The listing builds one solid part. Answer for the finished solid, in the listing's coordinates (mm). Face numbers are marked on the shaded views. A direction names the side the tool comes from. Round coordinates to 2 decimals unless told otherwise and drop trailing zeros. Loops run counter-clockwise (first coordinate to the right, second up) from the corner with the lowest first, then second, coordinate; pieces in that order, holes last. Notation, with made-up numbers: (42, 32) -> (54, 32) arc R19 ccw to (54, 57) -> close; hole circle Ø5 at (50, 56.25). An arc over 180 degrees is marked (long way). Answer in a Markdown table with one row per item. Add a question column.
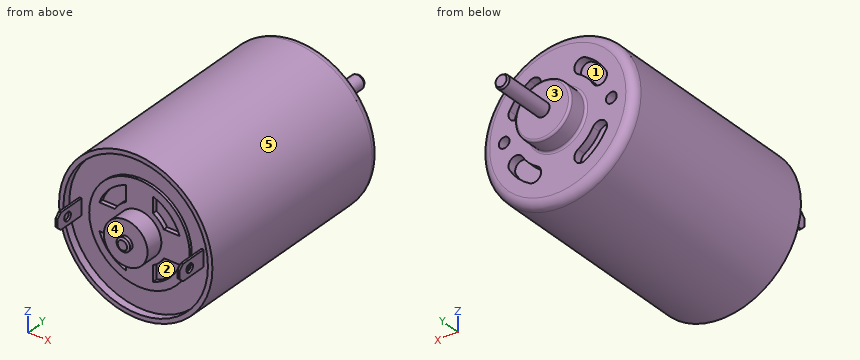
```python
from build123d import *
from OCP.BRepFilletAPI import BRepFilletAPI_MakeChamfer

# Parameters (mm, degrees)
SKETCH3_R          = 1.25
CUT_EXTRUDE2_DEPTH = 5
CUT_EXTRUDE3_DEPTH = 2
CIRPATTERN1_COUNT  = 4
CUT_EXTRUDE4_DEPTH = 1
CIRPATTERN2_COUNT  = 4
SKETCH6_W          = 3.8
SKETCH6_H          = 7.2
SKETCH6_R          = 1
EXTRUDE1_DEPTH     = 0.5
CHAMFER1_SIZE      = 1
FILLET1_R          = 2
FILLET3_R          = 0.5
CHAMFER2_SIZE      = 0.5
CHAMFER2_SIZE2     = 0.288675135


with BuildPart() as part:
    # Sketch1 → Revolve1 (revolve)
    with BuildSketch(Plane.XY, mode=Mode.PRIVATE) as revolve1_sk:
        Polygon((0, 42), (1.5875, 42), (1.5875, 29.5), (6.5, 29.5), (6.5, 25), (17.9, 25), (17.9, -25), (16.855, -25), (16.855, -23.25), (11.725, -23.25), (11.725, -23.87), (5.1, -23.87), (5.1, -28), (1.5875, -28), (1.5875, -29), (0, -29), align=None)
    revolve(revolve1_sk.sketch.rotate(Axis((0, 42, 0), (0, -1, 0)), 180), axis=Axis((0, 42, 0), (0, -1, 0)))

    # Sketch3 → Cut-Extrude2 (cut)
    with BuildSketch(Plane(origin=(0, 25, 0), x_dir=(1, 0, 0), z_dir=(0, 1, 0))):
        with Locations(Location((12.5, 0, 0), (0, 0, 180))):
            Circle(SKETCH3_R)
        with Locations((-12.5, 0)):
            Circle(SKETCH3_R)
    extrude(amount=-CUT_EXTRUDE2_DEPTH, mode=Mode.SUBTRACT)

    # Sketch4 → Cut-Extrude3 (cut)
    with BuildSketch(Plane(origin=(0, 25, 0), x_dir=(1, 0, 0), z_dir=(0, 1, 0))):
        with BuildLine():
            ThreePointArc((4.75, 8.227241336), (4.109455543, 10.617785793), (6.5, 11.258330249))
            Line((6.5, 11.258330249), (4.75, 8.227241336))
        make_face()
        with BuildLine():
            ThreePointArc((8.227241336, 4.75), (6.717514421, 6.717514421), (4.75, 8.227241336))
            Line((4.75, 8.227241336), (6.5, 11.258330249))
            ThreePointArc((6.5, 11.258330249), (9.192388155, 9.192388155), (11.258330249, 6.5))
            Line((11.258330249, 6.5), (8.227241336, 4.75))
        make_face()
        with BuildLine():
            Line((8.227241336, 4.75), (11.258330249, 6.5))
            ThreePointArc((11.258330249, 6.5), (10.617785793, 4.109455543), (8.227241336, 4.75))
        make_face()
    cut_extrude3 = extrude(amount=-CUT_EXTRUDE3_DEPTH, mode=Mode.SUBTRACT)

    # CirPattern1: Cut-Extrude3 ×4 about axis
    cirpattern1_axis = Axis((0, 0, 0), (0, 1, 0))
    for i in range(1, CIRPATTERN1_COUNT):
        add(cut_extrude3.rotate(cirpattern1_axis, i * 360 / CIRPATTERN1_COUNT), mode=Mode.SUBTRACT)

    # Sketch5 → Cut-Extrude4 (cut)
    with BuildSketch(Plane.XZ.offset(23.87)):
        with BuildLine():
            Line((3.15, 9.359119884), (3.15, 5.685727746))
            ThreePointArc((3.15, 5.685727746), (4.596194078, 4.596194078), (5.685727746, 3.15))
            Line((5.685727746, 3.15), (9.359119884, 3.15))
            ThreePointArc((9.359119884, 3.15), (6.982679464, 6.982679464), (3.15, 9.359119884))
        make_face()
    cut_extrude4 = extrude(amount=-CUT_EXTRUDE4_DEPTH, mode=Mode.SUBTRACT)

    # CirPattern2: Cut-Extrude4 ×4 about axis
    cirpattern2_axis = Axis((0, 0, 0), (0, 1, 0))
    for i in range(1, CIRPATTERN2_COUNT):
        add(cut_extrude4.rotate(cirpattern2_axis, i * 360 / CIRPATTERN2_COUNT), mode=Mode.SUBTRACT)

    # Sketch6 → Extrude1 (add)
    with BuildSketch(Plane(origin=(14, 0, 0), x_dir=(0, 0, -1), z_dir=(1, 0, 0))):
        with Locations((0, -26.85)):
            Rectangle(SKETCH6_W, SKETCH6_H)
        with Locations((0, -27.45)):
            Circle(SKETCH6_R, mode=Mode.SUBTRACT)
    extrude1 = extrude(amount=EXTRUDE1_DEPTH)

    # Mirror1: Extrude1 across plane
    add(extrude1.mirror(Plane(origin=(0, 0, 0), x_dir=(0, 0, 1), z_dir=(1, 0, 0))))

    # Chamfer1
    chamfer1_edges = [part.edges().sort_by_distance(p)[0] for p in [
        (14.25, -30.45, 1.9),
        (14.25, -30.45, -1.9),
        (-14.25, -30.45, 1.9),
        (-14.25, -30.45, -1.9),
    ]]
    chamfer(chamfer1_edges, length=CHAMFER1_SIZE)

    # Fillet1
    fillet1_edges = [part.edges().sort_by_distance(p)[0] for p in [
        (17.9, 25, 0),
    ]]
    fillet(fillet1_edges, radius=FILLET1_R)

    # Fillet3
    fillet3_edges = [part.edges().sort_by_distance(p)[0] for p in [
        (6.5, 25, 0),
        (6.5, 29.5, 0),
    ]]
    fillet(fillet3_edges, radius=FILLET3_R)

    # Chamfer2: one chamfer whose edges measure the first distance from different faces: ONE call of the kernel's chamfer builder (chamfer() names one face for all edges)
    chamfer2_edges_1 = [part.edges().sort_by_distance(p)[0] for p in [
        (1.5875, 42, 0),
    ]]
    chamfer2_side_1 = [part.faces().sort_by_distance(p)[0] for p in [
        (1.5875, 35.75, 0),
    ]]
    chamfer2_edges_2 = [part.edges().sort_by_distance(p)[0] for p in [
        (1.5875, -29, 0),
    ]]
    chamfer2_side_2 = [part.faces().sort_by_distance(p)[0] for p in [
        (0, -29, 0),
    ]]
    chamfer2 = BRepFilletAPI_MakeChamfer(part.part.solid().wrapped)
    for e in chamfer2_edges_1:
        chamfer2.Add(CHAMFER2_SIZE, CHAMFER2_SIZE2, e.wrapped, chamfer2_side_1[0].wrapped)  # the first distance lies on this face
    for e in chamfer2_edges_2:
        chamfer2.Add(CHAMFER2_SIZE, CHAMFER2_SIZE2, e.wrapped, chamfer2_side_2[0].wrapped)  # the first distance lies on this face
    add(Compound.cast(chamfer2.Shape()), mode=Mode.REPLACE)


solid = part.part
```
Item 1: Section A-A, the plane z = 0 is taken. Give the number of separate pieces and of enclosed holes in the cut face, and give its area (3 significant figures).
Item 2: Flat-ended cylindrical pins translate along their axes: P1, Ø3, axis at x = -12.5, z = 0, coming from the +Y side; P2, Ø10, axis at x = 5, z = -8.5, coming from the +Y side; P3, Ø12, axis at x = -3.5, y = -0.5, coming from the -Z side. Find the tip coordinate at first contact, or state that the pin passes through.
Item 3: Section B-B, the plane y = 10.5 is taken. Write down the section's boundary in (x, z), and give its area (3 significant figures).
Item 4: Consider L1, parallel to Z at x = 0, y = -24 (3 decimals); L2, parallel to Y at x = -14.3, z = 0; L3, parallel to Z at x = 1, y = 35.5. Determine where each line is inside the solid, lowest interval first. Write a range as from..to.
Item 5: The mould has two halves that part along X. Classify the marked faces 3, 4 and 5: +X half, -X half, draft (parallel to the pull), parting line (faces both ways), or undercut.
Item 6: For the marked faces 1 and 2, determine the directions among +Z, -Z, +X, -X, +Y, -Y from which every point of the face is accessible in a straight line to the end or side of a thin tool.
Here are the results:
| question | item | result |
|---|---|---|
| 1 | separate pieces | 3 |
| 1 | enclosed holes | 0 |
| 1 | area | 1,870 mm² |
| 2 | P1 | stops at y = 25 |
| 2 | P2 | stops at y = 29.5 |
| 2 | P3 | stops at z = -17.9 |
| 3 | outline | circle Ø35.8 at (0, 0) |
| 3 | area | 1,010 mm² |
| 4 | L1 | z = -17.9..-16.855, -5.1..5.1, 16.855..17.9 |
| 4 | L2 | y = -30.45..-28.45, -26.45..25 |
| 4 | L3 | z = -1.23..1.23 |
| 5 | face 3 | draft |
| 5 | face 4 | undercut |
| 5 | face 5 | parting line |
| 6 | face 1 | +Y |
| 6 | face 2 | -Y |
